Geometry: final body of the model. Coordinates: model frame, mm. Face numbers are marked on the shaded views. A direction names the side the tool comes from. Give positions to 0.01 mm unless a question says otherwise; leave off trailing zeros. Write each loop counter-clockwise with the first axis right and the second up, starting at its lowest first coordinate (ties: lowest second). Pieces come first, ordered by that corner, then holes.
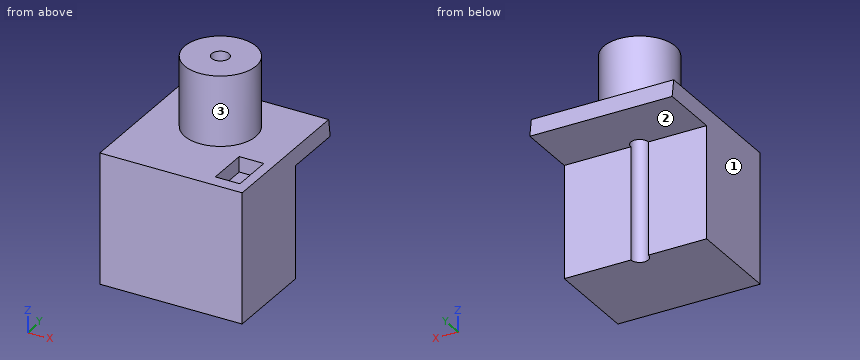
```python
from build123d import *

# Parameters (mm, degrees)
F1_DEPTH = 51.791012
F2_R     = 12.992445
F3_DEPTH = 25.4
F5_D     = 6.35
F6_W     = 8.970857
F6_H     = 15.168444
F7_DEPTH = 5.578703


with BuildPart() as f1:
    # F0 (on Right) → F1 (new body)
    with BuildSketch(Plane.YZ):
        Polygon((21.825537, 0), (20.848211, 6.495342), (-33.898331, 6.495342), (-33.898331, -40.874604), (0, -40.874604), (0, 0), align=None)
    extrude(amount=F1_DEPTH)

    # F2 (on face) → F3 (join)
    with BuildSketch(Plane.XY.offset(6.495342)):
        with Locations((24.38122, 0)):
            Circle(F2_R)
    extrude(amount=F3_DEPTH)

    # F5 (through all)
    with Locations(Plane.XY.offset(31.895342)):
        with Locations((24.38122, 0)):
            Hole(F5_D / 2)

    # F6 (on face) → F7 (cut)
    with BuildSketch(Plane.XY.offset(6.495342)):
        with Locations((43.771073, -21.581918)):
            Rectangle(F6_W, F6_H)
    extrude(amount=-F7_DEPTH, mode=Mode.SUBTRACT)


solid = f1.part
```
Item 1: Section C-C, the plane x = 5.5. Return the cut outline in (y, z).
Found:
outline: (-33.9, -40.87) - (0, -40.87) - (0, 0) - (21.83, 0) - (20.85, 6.5) - (-33.9, 6.5) - close
Item 2: Pin query (flat end, axial travel): pin 1 Ø3 at (x, z) = (31, -13) entering from +Y; pin 2 Ø7 at (x, y) = (42, -19.5) entering from +Z; pin 3 Ø2 at (y, z) = (-6, 13) entering from -X. Return the tip coordinate at first contact, or that it passes through.
Found:
pin 1: stops at y = 0
pin 2: stops at z = 6.5
pin 3: stops at x = 12.39
Item 3: Section B-B, the plane z = -26. Return the cut outline in (x, y) (3 decimals), plus the area to 3 significant figures.
Found:
outline: (0, -33.898) - (51.791, -33.898) - (51.791, 0) - (27.556, 0) arc R3.175 cw to (21.206, 0) - (0, 0) - close
area: 1,740 mm2
Item 4: Reachability of the marked faces 1, 2 and 3 from +Z, -Z, +X, -X, +Y, -Y: full face, straight path, thin tool, end or side. Return the list, or none.
Found:
face 1: +Z, -Z, -X, +Y, -Y
face 2: -Z, +X, -X, +Y
face 3: +Z
Item 5: Section A-A, the plane y = -16. Return the cut outline in (x, z).
Found:
outline: (0, -40.87) - (51.79, -40.87) - (51.79, 6.5) - (48.26, 6.5) - (48.26, 0.92) - (39.29, 0.92) - (39.29, 6.5) - (0, 6.5) - close
Item 6: Section D-D, the plane z = 3. State how many separate pieces and enclosed holes the cut face has, plus the area to 3 significant figures.
Found:
separate pieces: 1
enclosed holes: 2
area: 2,690 mm2
Item 7: Line query: L1, parallel to Z at x = 42.5, y = -15; L2, parallel to Y at x = 38.5, z = -26; L3, parallel to Z at x = 8, y = 18.5. Output: solid intervals per line, ascending.
Found:
L1: z = -40.87 to 0.92
L2: y = -33.9 to 0
L3: z = 0 to 6.5
